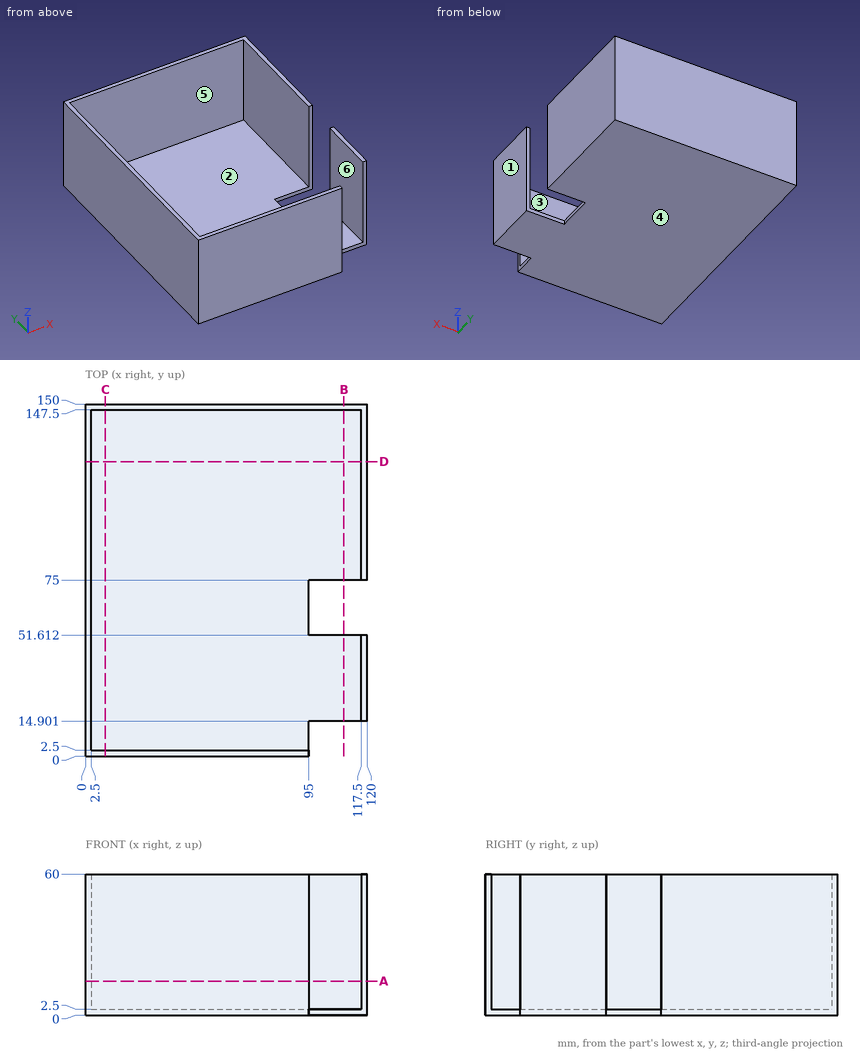
Print and shaded views of the part. All mm, measured from the part's lowest x, y and z. A direction names the side the tool comes from. Coordinates: 2 decimals unless noted, no trailing zeros. Loops run counter-clockwise (first coordinate to the right, second up) from the corner with the lowest first, then second, coordinate; pieces in that order, holes last. Notation, with made-up numbers: (86.25, -11.5) - (96.25, -11.5) arc R20 cw to (96.25, 10.5) - close; hole circle Ø6 at (-30, 6.5). An arc over 180 degrees is marked (long way). Write item = value, one per line. Start each with the question number.
Item 1: Pull direction X, two halves, no side cores. Call the marked faces 1, 2 and 3: +X half, -X half, draft (parallel to the pull), parting line (faces both ways), or undercut.
Item 2: Saw through at B-B, the plane x = 110. List the corners of the cut face in (y, z), then the cut area to 3 significant figures.
Item 3: Saw through at A-A, the plane z = 14.5. List the corners of the cut face in (x, y).
Item 4: Wall check: probe 1 along X at (y, z) = (91, 25); probe 2 along Y at (x, z) = (73, 17); probe 3 along Z at (x, y) = (64.5, 113). Give the ranges that are in metal, low to high. Write a range as [from, to].
Item 5: Drop flat-ended pins along their axis: pin 1 Ø20 at (x, z) = (111.5, 28.5) entering from -Y; pin 2 Ø10 at (x, y) = (97, 130) entering from +Z; pin 3 Ø2 at (y, z) = (67, 1.5) entering from +X. Give the stop position or say it passes through.
Item 6: Saw through at D-D, the plane y = 125.5. List the corners of the cut face in (x, z).
Item 7: Saw through at C-C, the plane x = 8.5. List the corners of the cut face in (y, z).
Item 8: 3-axis set-ups, long thin cutter, end or side, ignore diameter. For the marked faces 4, 5 and 6: which of +Z, -Z, +X, -X, +Y, -Y reach the whole face in a straight line?
Answers:
q1.face_1 = +X half
q1.face_2 = undercut
q1.face_3 = draft
q2.outline = (14.9, 0) - (51.61, 0) - (51.61, 2.5) - (14.9, 2.5) - close; (75, 0) - (150, 0) - (150, 60) - (147.5, 60) - (147.5, 2.5) - (75, 2.5) - close
q2.area = 423 mm2
q3.outline = (0, 0) - (95, 0) - (95, 2.5) - (2.5, 2.5) - (2.5, 147.5) - (117.5, 147.5) - (117.5, 75) - (120, 75) - (120, 150) - (0, 150) - close; (117.5, 14.9) - (120, 14.9) - (120, 51.61) - (117.5, 51.61) - close
q4.probe_1 = [0, 2.5], [117.5, 120]
q4.probe_2 = [0, 2.5], [147.5, 150]
q4.probe_3 = [0, 2.5]
q5.pin_1 = 14.9
q5.pin_2 = 2.5
q5.pin_3 = 95
q6.outline = (0, 0) - (120, 0) - (120, 60) - (117.5, 60) - (117.5, 2.5) - (2.5, 2.5) - (2.5, 60) - (0, 60) - close
q7.outline = (0, 0) - (150, 0) - (150, 60) - (147.5, 60) - (147.5, 2.5) - (2.5, 2.5) - (2.5, 60) - (0, 60) - close
q8.face_4 = -Z, +X, -X, +Y, -Y
q8.face_5 = +Z
q8.face_6 = +Z, -Y
